For this review, use the dimensioned drawing (mm, ordinates from the lowest corner) and the shaded views. Coordinates: 2 decimals unless noted, no trailing zeros. Write each loop counter-clockwise with the first axis right and the second up, starting at its lowest first coordinate (ties: lowest second). Pieces come first, ordered by that corner, then holes.
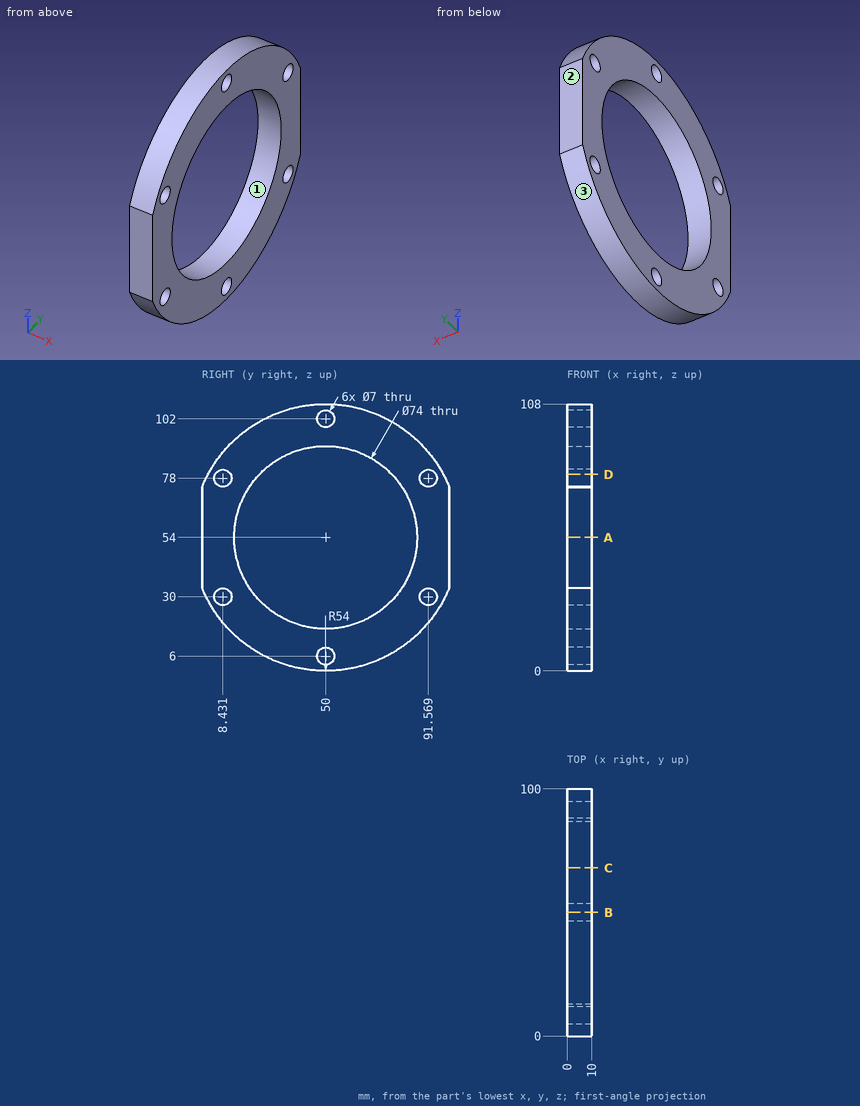
(1) Consider section C-C (y = 68). Give the boundary of the cut face in (x, z).
(2) Consider section B-B (y = 50). Give the boundary of the cut face in (x, z), plus the area to 3 significant figures.
(3) Mouldability with a two-part tool opening along Z and no side actions: class the marked faces 1, 2 and 3 as +Z half, -Z half, draft (parallel to the pull), parting line (faces both ways), or undercut.
(4) Insertion check: pin 1 Ø4 at (x, y) = (2.5, 49) entering from -Z; pin 2 Ø1.5 at (x, y) = (6, 43.5) entering from -Z; pin 3 Ø2 at (x, z) = (9, 18.5) entering from -Y. Each pin has a flat end and moves straight along its axis. Give the tip position at first contact, or say it passes through.
(5) Consider section A-A (z = 54). Give the boundary of the cut face in (x, y).
(6) Wall thickness on line 1 (Z direction, x = 7.5, y = 50.5); line 2 (Z direction, x = 3.25, y = 94.5) (1 decimal); line 3 (Z direction, x = 7, y = 34) (1 decimal): over which ranges is each line inside the solid? List them lowest first.
(7) Consider section D-D (z = 79.5). Give the boundary of the cut face in (x, y), plus the area to 3 significant figures.
Results:
1. outline: (0, 3.09) - (10, 3.09) - (10, 21.67) - (0, 21.67) - close; (0, 86.33) - (10, 86.33) - (10, 104.91) - (0, 104.91) - close
2. outline: (0, 0) - (10, 0) - (10, 2.5) - (0, 2.5) - close; (0, 9.5) - (10, 9.5) - (10, 17) - (0, 17) - close; (0, 91) - (10, 91) - (10, 98.5) - (0, 98.5) - close; (0, 105.5) - (10, 105.5) - (10, 108) - (0, 108) - close
2. area: 200 mm2
3. face 1: undercut
3. face 2: draft
3. face 3: -Z half
4. pin 1: stops at z = 0
4. pin 2: stops at z = 0.31
4. pin 3: stops at y = 8.46
5. outline: (0, 0) - (10, 0) - (10, 13) - (0, 13) - close; (0, 87) - (10, 87) - (10, 100) - (0, 100) - close
6. line 1: z = 0 to 2.54, 9.46 to 17, 91 to 98.54, 105.46 to 108
6. line 2: z = 23.4 to 28.1, 31.9 to 76.1, 79.9 to 84.6
6. line 3: z = 2.4 to 20.6, 87.4 to 105.6
7. outline: (0, 2.4) - (10, 2.4) - (10, 5.27) - (0, 5.27) - close; (0, 11.59) - (10, 11.59) - (10, 23.19) - (0, 23.19) - close; (0, 76.81) - (10, 76.81) - (10, 88.41) - (0, 88.41) - close; (0, 94.73) - (10, 94.73) - (10, 97.6) - (0, 97.6) - close
7. area: 289 mm2
